Verification items for the finished model (mm, model axes). Face numbers are marked on the shaded views. A direction names the side the tool comes from. Round coordinates to 2 decimals unless told otherwise and drop trailing zeros. Answer as a JSON object with one key per item and string values. Group by question number.
```python
from build123d import *

# Parameters (mm, degrees)
SKETCH1_R           = 24.60625
SKETCH1_R_2         = 3.175
BOSS_EXTRUDE1_DEPTH = 15.875
SKETCH2_R           = 12.7
SKETCH2_R_2         = 9.525
CUT_EXTRUDE1_DEPTH  = 6.35
CUT_EXTRUDE3_START  = -6.35
SKETCH4_R           = 12.7
SKETCH4_R_2         = 9.525
CUT_EXTRUDE3_DEPTH  = 6.35
CHAMFER1_SIZE       = 3.175
CHAMFER1_SIZE2      = 6.35
CHAMFER2_SIZE       = 6.35
CHAMFER2_SIZE2      = 3.175
CUT_EXTRUDE5_DEPTH  = 39.248538575
CIRPATTERN2_COUNT   = 8
SKETCH6_R           = 1.27
BOSS_EXTRUDE2_DEPTH = 6.35
SKETCH9_R           = 1.27
BOSS_EXTRUDE3_DEPTH = 6.35
CUT_EXTRUDE6_REACH  = 43.528
CIRPATTERN3_COUNT   = 8
SKETCH16_W          = 12.7
SKETCH16_H          = 9.525
CUT_EXTRUDE7_DEPTH  = 6.35
CIRPATTERN4_COUNT   = 8


with BuildPart() as part:
    # Sketch1 → Boss-Extrude1 (new body)
    with BuildSketch(Plane.XY):
        Circle(SKETCH1_R)
        Circle(SKETCH1_R_2, mode=Mode.SUBTRACT)
    extrude(amount=BOSS_EXTRUDE1_DEPTH)

    # Sketch2 → Cut-Extrude1 (cut)
    with BuildSketch(Plane.XY.offset(15.875)):
        Circle(SKETCH2_R)
        Circle(SKETCH2_R_2, mode=Mode.SUBTRACT)
    extrude(amount=-CUT_EXTRUDE1_DEPTH, mode=Mode.SUBTRACT)

    # Sketch4 → Cut-Extrude3 (cut)
    with BuildSketch(Plane(origin=(0, 0, 0), x_dir=(-1, 0, 0), z_dir=(0, 0, -1)).offset(CUT_EXTRUDE3_START)):
        with Locations(Location((0, 0, 0), (0, 0, 180))):
            Circle(SKETCH4_R)
        with Locations(Location((0, 0, 0), (0, 0, 180))):
            Circle(SKETCH4_R_2, mode=Mode.SUBTRACT)
    extrude(amount=CUT_EXTRUDE3_DEPTH, mode=Mode.SUBTRACT)

    # Chamfer1
    chamfer1_edges = [part.edges().sort_by_distance(p)[0] for p in [
        (-24.60625, 0, 0),
    ]]
    chamfer1_side = [part.faces().sort_by_distance(p)[0] for p in [
        (-23.910280151, 0, 0),
    ]]
    chamfer(chamfer1_edges, length=CHAMFER1_SIZE, length2=CHAMFER1_SIZE2, reference=chamfer1_side[0])

    # Chamfer2
    chamfer2_edges = [part.edges().sort_by_distance(p)[0] for p in [
        (-24.60625, 0, 15.875),
    ]]
    chamfer2_side = [part.faces().sort_by_distance(p)[0] for p in [
        (-24.60625, 0, 11.1125),
    ]]
    chamfer(chamfer2_edges, length=CHAMFER2_SIZE, length2=CHAMFER2_SIZE2, reference=chamfer2_side[0])

    # Sketch5 → Cut-Extrude5 (cut, through all)
    with BuildSketch(Plane(origin=(0, 0, 0), x_dir=(-1, 0, 0), z_dir=(0, 0, -1))):
        with BuildLine():
            Line((-6.35, 26.286223353), (6.35, 26.286223353))
            Line((6.35, 26.286223353), (6.35, 22.125558785))
            ThreePointArc((6.35, 22.125558785), (0, 23.01875), (-6.35, 22.125558785))
            Line((-6.35, 22.125558785), (-6.35, 26.286223353))
        make_face()
    cut_extrude5 = extrude(amount=-CUT_EXTRUDE5_DEPTH, mode=Mode.SUBTRACT)

    # CirPattern2: Cut-Extrude5 ×8 about axis
    cirpattern2_axis = Axis((0, 0, 0), (0, 0, 1))
    for i in range(1, CIRPATTERN2_COUNT):
        add(cut_extrude5.rotate(cirpattern2_axis, i * 360 / CIRPATTERN2_COUNT), mode=Mode.SUBTRACT)

    # Sketch6 → Boss-Extrude2 (add)
    with BuildSketch(Plane(origin=(0, 0, 6.35), x_dir=(-1, 0, 0), z_dir=(0, 0, -1))):
        with Locations((0, -11.1125)):
            Circle(SKETCH6_R)
    extrude(amount=BOSS_EXTRUDE2_DEPTH)

    # Sketch9 → Boss-Extrude3 (add)
    with BuildSketch(Plane.XY.offset(9.525)):
        with Locations((0, 11.1125)):
            Circle(SKETCH9_R)
    extrude(amount=BOSS_EXTRUDE3_DEPTH)

    # Sketch14 → Cut-Extrude6 (cut, up to next)
    with BuildSketch(Plane.ZY.offset(-6.35), mode=Mode.PRIVATE) as cut_extrude6_sk1:
        Polygon((6.35, 23.772779372), (9.525, 23.772779372), (12.7, 22.125558785), (3.175, 22.125558785), align=None)
    cut_extrude6_tool1 = extrude(cut_extrude6_sk1.sketch, amount=CUT_EXTRUDE6_REACH, mode=Mode.PRIVATE) & part.part
    cut_extrude6 = cut_extrude6_tool1.solids().sort_by_distance((6.35, 22.811901, 7.9375))[0]
    add(cut_extrude6, mode=Mode.SUBTRACT)

    # CirPattern3: Cut-Extrude6 ×8 about axis
    cirpattern3_axis = Axis((0, 0, 0), (0, 0, 1))
    for i in range(1, CIRPATTERN3_COUNT):
        add(cut_extrude6.rotate(cirpattern3_axis, i * 360 / CIRPATTERN3_COUNT), mode=Mode.SUBTRACT)

    # Sketch16 → Cut-Extrude7 (cut, symmetric)
    with BuildSketch(Plane(origin=(0, 22.125558785, 0), x_dir=(1, 0, 0), z_dir=(0, 1, 0))):
        with Locations((0, -7.9375)):
            Rectangle(SKETCH16_W, SKETCH16_H)
    cut_extrude7 = extrude(amount=CUT_EXTRUDE7_DEPTH, both=True, mode=Mode.SUBTRACT)

    # CirPattern4: Cut-Extrude7 ×8 about axis
    cirpattern4_axis = Axis((0, 0, 0), (0, 0, 1))
    for i in range(1, CIRPATTERN4_COUNT):
        add(cut_extrude7.rotate(cirpattern4_axis, i * 360 / CIRPATTERN4_COUNT), mode=Mode.SUBTRACT)


solid = part.part
```
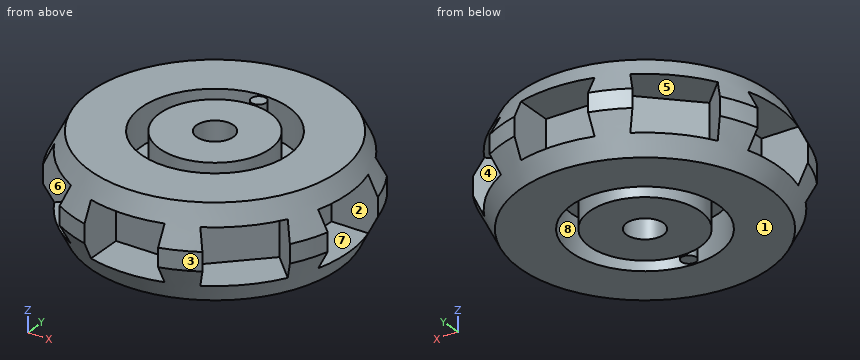
Q1. Gauge pin test, flat ends, axial feed: pin 1 Ø4 at (x, z) = (-10, 6) entering from +Y; pin 2 Ø2 at (x, z) = (-12.5, 10) entering from +Y; pin 3 Ø2.5 at (y, z) = (18.5, 7.5) entering from -X. Record the tip position at first contact, or that the pin passes through.
Q2. Release check for a two-part mould opening along Y. For the marked faces 1, 2 and 3 record: released by +Y, released by -Y, zero draft, split by the parting line, or undercut.
Q3. Cross-section at B-B, the plane z = 13.5. Give the number of separate pieces and of enclosed holes in the cut face, then the cut area to 3 significant figures.
Q4. Tool access check on the marked faces 4, 5, 6, 7 and 8. Record the directions out of +Z, -Z, +X, -X, +Y, -Y that give a thin tool (end or side, any length) a straight path to the whole face; none if there is none.
Q5. Thickness scan on line 1 (Y direction, x = 0, z = 3.5) (1 decimal); line 2 (Y direction, x = 0, z = 11) (1 decimal); line 3 (Y direction, x = 0, z = 8.5) (3 decimals). Record the ranges inside material, lowest first. Write a range as from..to.
Conclusion:
{
 "1": {"pin 1": "y = 23.26", "pin 2": "y = 21.69", "pin 3": "x = -10.77"},
 "2": {"face 1": "zero draft", "face 2": "undercut", "face 3": "released by -Y"},
 "3": {"separate pieces": "3", "enclosed holes": "2", "area": "1,360 mm2"},
 "4": {"face 4": "+Y", "face 5": "none", "face 6": "-Y", "face 7": "+X", "face 8": "-Z"},
 "5": {"line 1": "-15.8..-12.7, -12.4..-9.8, -9.5..-3.2, 3.2..9.5, 12.7..15.8", "line 2": "-15.8..-12.7, -9.5..-3.2, 3.2..9.5, 9.8..12.4, 12.7..15.8", "line 3": "-15.776..-3.175, 3.175..15.776"}
}
